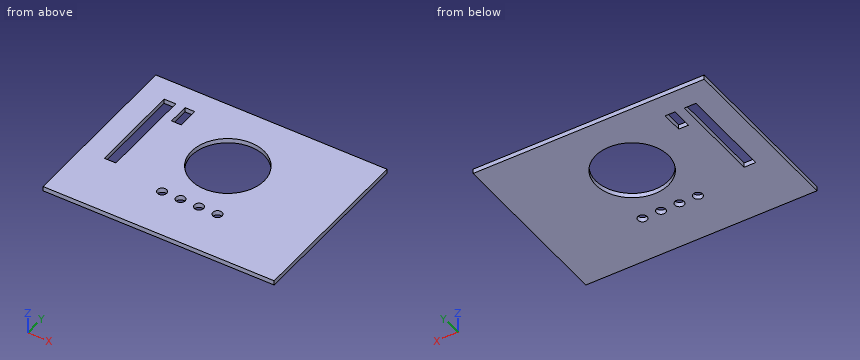
Autodesk Inventor part; units mm, degrees
ref_plane "YZ Plane" through (0, 0, 0) normal (1, 0, 0) x (0, 1, 0)
ref_plane "XZ Plane" through (0, 0, 0) normal (0, 1, 0) x (-1, 0, 0)
ref_plane "XY Plane" through (0, 0, 0) normal (0, 0, 1) x (1, 0, 0)
sketch "Sketch1" plane through (0, 0, 0) normal (0, 0, 1) x (1, 0, 0)
  line L0 (-317.5, 241.3) -> (0, 241.3)
  line L1 (0, 241.3) -> (0, 0)
  line L2 (0, 0) -> (-317.5, 0)
  line L3 (-317.5, 0) -> (-317.5, 241.3)
  dimension "d0" = 317.5
  dimension "d1" = 241.3
extrude "Extrusion1" add sketch "Sketch1" along normal blind 6.35
sketch "Sketch2" plane through (0, 0, 6.35) normal (0, 0, 1) x (1, 0, 0)
  circle A0 centre (-120.65, 66.675) radius 6.35
  line L0 (-317.5, 0) -> (0, 0)
  line L1 (0, 0) -> (0, 241.3)
  circle A1 centre (-196.85, 66.675) radius 6.35
  line L2 (-317.5, 241.3) -> (-317.5, 0)
  circle A2 centre (-171.45, 66.675) radius 6.35
  circle A3 centre (-146.05, 66.675) radius 6.35
  dimension "d4" = 12.7
  dimension "d5" = 66.675
  dimension "d7" = 12.7
  dimension "d8" = 66.675
  dimension "d10" = 12.7
  dimension "d11" = 12.7
  dimension "d12" = 66.675
  dimension "d13" = 66.675
  dimension "d20" = 114.3
  dimension "d21" = 114.3
  dimension "d26" = 12.7
  dimension "d27" = 12.7
extrude "Extrusion2" cut sketch "Sketch2" against normal blind 6.35
sketch "Sketch3" plane through (0, 0, 6.35) normal (0, 0, 1) x (1, 0, 0)
  circle A0 centre (-157.9499, 146.8501) radius 49.9999
  line L0 (0, 0) -> (0, 241.3)
  line L1 (0, 241.3) -> (-317.5, 241.3)
  dimension "d28" = 99.9998
  dimension "d29" = 107.95
  dimension "d30" = 44.45
extrude "Extrusion3" cut sketch "Sketch3" against normal blind 6.35
sketch "Sketch4" plane through (0, 0, 6.35) normal (0, 0, 1) x (1, 0, 0)
  line L0 (-285.75, 209.55) -> (-269.748, 209.55)
  line L1 (-269.748, 209.55) -> (-269.748, 81.5594)
  line L2 (-269.748, 81.5594) -> (-285.75, 81.5594)
  line L3 (-285.75, 81.5594) -> (-285.75, 209.55)
  line L4 (-317.5, 241.3) -> (-317.5, 0)
  line L5 (0, 241.3) -> (-317.5, 241.3)
  point P0 (0, 0)
  dimension "d33" = 31.75
  dimension "d34" = 31.75
  dimension "d35" = 16.002
  dimension "d36" = 127.9906
extrude "Extrusion4" cut sketch "Sketch4" against normal blind 6.35
sketch "Sketch5" plane through (0, 0, 6.35) normal (0, 0, 1) x (1, 0, 0)
  line L0 (-257.048, 209.55) -> (-243.6368, 209.55)
  line L1 (-243.6368, 209.55) -> (-243.6368, 180.7464)
  line L2 (-243.6368, 180.7464) -> (-257.048, 180.7464)
  line L3 (-257.048, 180.7464) -> (-257.048, 209.55)
  line L4 (-269.748, 209.55) -> (-269.748, 81.5594)
  line L5 (0, 241.3) -> (-317.5, 241.3)
  point P0 (0, 0)
  dimension "d39" = 12.7
  dimension "d40" = 31.75
  dimension "d41" = 13.4112
  dimension "d42" = 28.8036
extrude "Extrusion5" cut sketch "Sketch5" against normal blind 6.35
properties part number "Base"
For this review, take the finished solid that the model builds, in its own axes (mm). Coordinates: 2 decimals unless noted, no trailing zeros. Loops run counter-clockwise (first coordinate to the right, second up) from the corner with the lowest first, then second, coordinate; pieces in that order, holes last. Notation, with made-up numbers: (-13, 31.25) -> (36, 31.25) arc R21 ccw to (36, 50.25) -> close; hole circle Ø6 at (84.5, 87). An arc over 180 degrees is marked (long way). Return JSON: item names as keys, results as strings. Group by question number.
(1) To check wall thickness, follow L1, parallel to Y at x = -274, z = 4; L2, parallel to X at y = 102, z = 0.75; L3, parallel to X at y = 67, z = 1. State the ranges of each line that lie inside material, in increasing order.
(2) For pin 1 Ø7.5 at (x, y) = (-120.65, 66.675) entering from -Z, flat-tipped, find the tip position at first contact; note if it passes through.
(3) Consider section C-C, the plane z = 4.25. Give the boundary of the cut face in (x, y) (3 decimals).
(4) Consider section B-B, the plane x = -196.85. Give the boundary of the cut face in (y, z) (3 decimals), plus the area to 3 significant figures.
(5) Consider section A-A, the plane y = 162.5. Give the boundary of the cut face in (x, z).
Results below:
{
 "1": {"L1": "y = 0 to 81.56, 209.55 to 241.3", "L2": "x = -317.5 to -285.75, -269.75 to -180.05, -135.85 to 0", "L3": "x = -317.5 to -203.19, -190.51 to -177.79, -165.11 to -152.39, -139.71 to -126.99, -114.31 to 0"},
 "2": {"pin 1": "passes through"},
 "3": {"outline": "(-317.5, 0) -> (0, 0) -> (0, 241.3) -> (-317.5, 241.3) -> close; hole (-285.75, 81.559) -> (-269.748, 81.559) -> (-269.748, 209.55) -> (-285.75, 209.55) -> close; hole (-257.048, 180.746) -> (-243.637, 180.746) -> (-243.637, 209.55) -> (-257.048, 209.55) -> close; hole circle Ø100 at (-157.95, 146.85); hole circle Ø12.7 at (-196.85, 66.675); hole circle Ø12.7 at (-171.45, 66.675); hole circle Ø12.7 at (-146.05, 66.675); hole circle Ø12.7 at (-120.65, 66.675)"},
 "4": {"outline": "(0, 0) -> (60.325, 0) -> (60.325, 6.35) -> (0, 6.35) -> close; (73.025, 0) -> (115.437, 0) -> (115.437, 6.35) -> (73.025, 6.35) -> close; (178.263, 0) -> (241.3, 0) -> (241.3, 6.35) -> (178.263, 6.35) -> close", "area": "1,050 mm2"},
 "5": {"outline": "(-317.5, 0) -> (-285.75, 0) -> (-285.75, 6.35) -> (-317.5, 6.35) -> close; (-269.75, 0) -> (-205.44, 0) -> (-205.44, 6.35) -> (-269.75, 6.35) -> close; (-110.46, 0) -> (0, 0) -> (0, 6.35) -> (-110.46, 6.35) -> close"}
}
